```python
from build123d import *

# Parameters (mm, degrees)
F0_W     = 2260.6
F0_H     = 114.3
F1_DEPTH = 1968.5
F2_W     = 711.2
F2_H     = 1828.8
F3_DEPTH = 114.301
F4_W     = 196.85
F4_H     = 222.25
F5_DEPTH = 114.301


with BuildPart() as f1:
    # F0 (on Top) → F1 (new body)
    with BuildSketch(Plane.XY):
        with Locations((-1130.3, -971.55)):
            Rectangle(F0_W, F0_H)
    extrude(amount=F1_DEPTH)

    # F2 (on face) → F3 (cut, through all)
    with BuildSketch(Plane.XZ.offset(1028.7)):
        with Locations((-1092.2, 914.4)):
            Rectangle(F2_W, F2_H)
    extrude(amount=-F3_DEPTH, mode=Mode.SUBTRACT)

    # F4 (on face) → F5 (cut, through all)
    with BuildSketch(Plane.XZ.offset(1028.7)):
        with Locations((-2162.175, 111.125)):
            Rectangle(F4_W, F4_H)
        with Locations((-98.425, 111.125)):
            Rectangle(F4_W, F4_H)
    extrude(amount=-F5_DEPTH, mode=Mode.SUBTRACT)


solid = f1.part
```
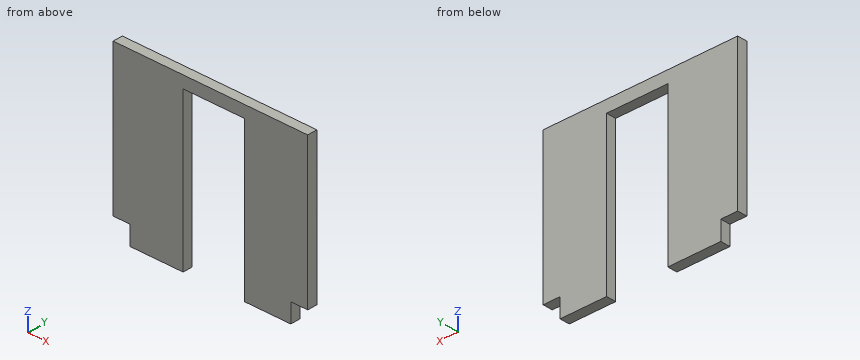
Design review of the part built by this model. Coordinates are the model's own, in mm. Coordinates: 2 decimals unless noted, no trailing zeros. Order: outer loops, then holes, each group sorted by start corner. A loop starts at its lowest first (then second) coordinate and runs counter-clockwise, first axis right, second up. Notation, with made-up numbers: (39, 4) - (73, 4) arc R28 cw to (73, 24) - close; hole circle Ø6 at (56, 47.5). An arc over 180 degrees is marked (long way). Answer in a Markdown table with one row per item.
(1) Clearance check with flat-ended pins moving along their axes: pin 1 (1 mm diameter, centred on y = -963, z = 1391.5, fed in from +X); pin 2 (8 mm diameter, centred on y = -997.5, z = 209.5, fed in from -X). State where each tip first meets the part, or that it passes through.
Checked values:
| item | result |
|---|---|
| pin 1 | x = 0 |
| pin 2 | x = -2063.75 |
(2) Wall thickness on line 1 along X through (y, z) = (-980, 250); line 2 along X through (y, z) = (-975, 96.5); line 3 along Z through (x, y) = (-926.5, -981): over which ranges is each line inside the solid? List them lowest first. Write a range as from..to.
Checked values:
| item | result |
|---|---|
| line 1 | -2260.6..-1447.8, -736.6..0 |
| line 2 | -2063.75..-1447.8, -736.6..-196.85 |
| line 3 | 1828.8..1968.5 |
(3) Consider section C-C on x = -1214. State the section outline as (y, z) points, plus the area to 3 significant figures.
Checked values:
| item | result |
|---|---|
| outline | (-1028.7, 1828.8) - (-914.4, 1828.8) - (-914.4, 1968.5) - (-1028.7, 1968.5) - close |
| area | 16,000 mm^2 |
(4) Consider section B-B on y = -1007.5. State the section outline as (x, z) points.
Checked values:
| item | result |
|---|---|
| outline | (-2260.6, 222.25) - (-2063.75, 222.25) - (-2063.75, 0) - (-1447.8, 0) - (-1447.8, 1828.8) - (-736.6, 1828.8) - (-736.6, 0) - (-196.85, 0) - (-196.85, 222.25) - (0, 222.25) - (0, 1968.5) - (-2260.6, 1968.5) - close |
(5) Consider section D-D on x = -164. State the section outline as (y, z) points, plus the area to 3 significant figures.
Checked values:
| item | result |
|---|---|
| outline | (-1028.7, 222.25) - (-914.4, 222.25) - (-914.4, 1968.5) - (-1028.7, 1968.5) - close |
| area | 200,000 mm^2 |
(6) Consider section A-A on z = 1712.5. State the section outline as (x, y) points, plus the area to 3 significant figures.
Checked values:
| item | result |
|---|---|
| outline | (-2260.6, -1028.7) - (-1447.8, -1028.7) - (-1447.8, -914.4) - (-2260.6, -914.4) - close; (-736.6, -1028.7) - (0, -1028.7) - (0, -914.4) - (-736.6, -914.4) - close |
| area | 177,000 mm^2 |
